```python
from build123d import *

# Parameters (mm, degrees)
F2_R     = 10.411054
F3_DEPTH = 47.962751
F4_R     = 1.524
F5_R     = 1.524


with BuildPart() as f1:
    # F0 (on Front) → F1 (revolve)
    with BuildSketch(Plane.XZ):
        Polygon((-35.411011, 28.463284), (-35.411011, 14.567823), (36.755737, 14.567823), (36.755737, 28.463284), (12.55074, 28.463284), (12.55074, 94.802901), (-10.757774, 94.802901), (-10.757774, 28.463284), align=None)
    revolve(axis=Axis((-25.101472, 0, 0), (1, 0, 0)))

    # F2 (on face) → F3 (cut, through all)
    with BuildSketch(Plane.YZ.offset(12.55074)):
        with Locations((0, 65.46654)):
            Circle(F2_R)
        with Locations((-46.291835, 46.291835)):
            Circle(F2_R)
        with Locations((-65.46654, 0)):
            Circle(F2_R)
        with Locations((-46.291835, -46.291835)):
            Circle(F2_R)
        with Locations((0, -65.46654)):
            Circle(F2_R)
        with Locations((46.291835, -46.291835)):
            Circle(F2_R)
        with Locations((65.46654, 0)):
            Circle(F2_R)
        with Locations((46.291835, 46.291835)):
            Circle(F2_R)
    extrude(amount=-F3_DEPTH, mode=Mode.SUBTRACT)

    # F4
    f4_edges = [f1.edges().sort_by_distance(p)[0] for p in [
        (-10.757774, 0, -94.802901),
    ]]
    fillet(f4_edges, radius=F4_R)

    # F5
    f5_edges = [f1.edges().sort_by_distance(p)[0] for p in [
        (12.55074, 0, -94.802901),
        (36.755737, 0, -28.463284),
        (-35.411011, 0, -28.463284),
    ]]
    fillet(f5_edges, radius=F5_R)


solid = f1.part
```
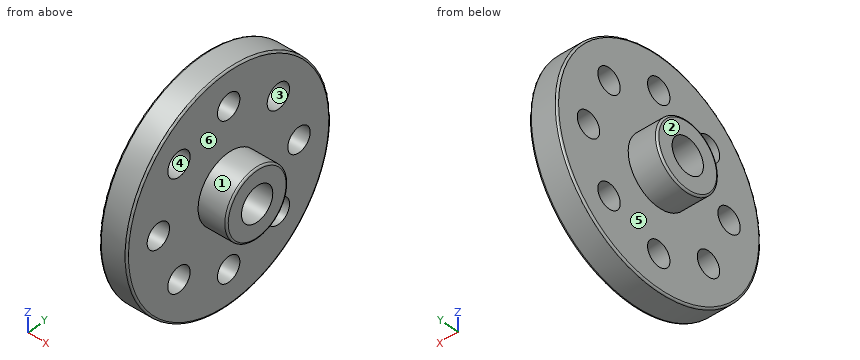
The model under review builds one solid part; all positions refer to its coordinate system, in mm. Face numbers are marked on the shaded views. A direction names the side the tool comes from. Round coordinates to 2 decimals unless told otherwise and drop trailing zeros. Order: outer loops, then holes, each group sorted by start corner. A loop starts at its lowest first (then second) coordinate and runs counter-clockwise, first axis right, second up. Notation, with made-up numbers: (74.5, 8) -> (110.5, 8) arc R11 ccw to (110.5, 28) -> close; hole circle Ø7 at (-4.75, -35). An arc over 180 degrees is marked (long way). One line per item, written item: value. Start each with the question number.
Q1. Take a section at C-C (x = 28). Write out the cut boundary in (y, z).
Q2. Clearance check with flat-ended pins moving along their axes: pin 1 Ø6 at (x, z) = (10, 64.5) entering from +Y; pin 2 Ø6 at (x, z) = (-11, 25) entering from -Y; pin 3 Ø3 at (x, z) = (-11.5, 2) entering from -Y. State where each tip first meets the part, or that it passes through.
Q3. Wall thickness on line 1 (Z direction, x = 1, y = 0); line 2 (Y direction, x = -10, z = -45); line 3 (Y direction, x = 17, z = 0): over which ranges is each line inside the solid? List them lowest first.
Q4. Take a section at A-A (z = 0). Count the separate pieces of the cut face and the enclosed holes in it, and give its area (3 significant figures).
Q5. Mouldability with a two-part tool opening along Y and no side actions: class the marked faces 1, 2 and 3 as released by +Y, released by -Y, zero draft, split by the parting line, or undercut.
Q6. Machinability: for the marked faces 4, 5 and 6, which of the approach directions +Z, -Z, +X, -X, +Y, -Y give a long, thin tool a straight path to every point of the face, cutting with its end or side? Answer none if there is none.
Reported:
1. outline: circle Ø56.93 at (0, 0); hole circle Ø29.14 at (0, 0)
2. pin 1: stops at y = 72.15
2. pin 2: stops at y = -92.1
2. pin 3: stops at y = -94.58
3. line 1: z = -94.8 to -75.88, -55.06 to -14.57, 14.57 to 55.06, 75.88 to 94.8
3. line 2: y = -83.21 to -56.62, -35.96 to 35.96, 56.62 to 83.21
3. line 3: y = -28.46 to -14.57, 14.57 to 28.46
4. separate pieces: 4
4. enclosed holes: 0
4. area: 4,120 mm2
5. face 1: split by the parting line
5. face 2: zero draft
5. face 3: undercut
6. face 4: +X, -X
6. face 5: -X
6. face 6: +X
